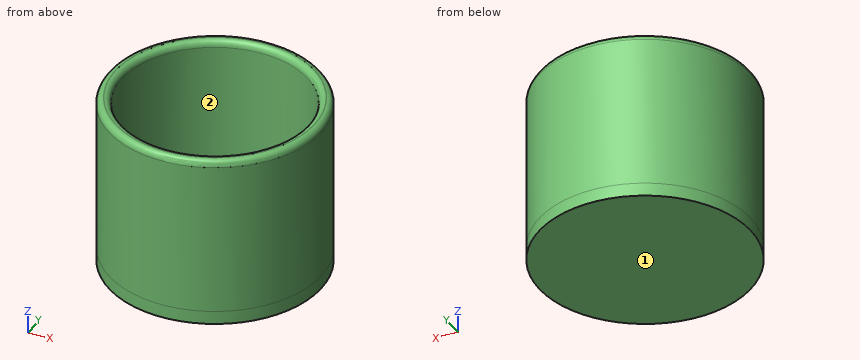
from build123d import *

# Parameters (mm, degrees)
F0_R     = 50.8
F1_DEPTH = 6.35
F2_R     = 50.8
F2_R_2   = 44.45
F3_DEPTH = 76.2
F4_R     = 3.066051
F5_R     = 3.066051


with BuildPart() as f1:
    # F0 (on Top) → F1 (new body)
    with BuildSketch(Plane.XY):
        Circle(F0_R)
    extrude(amount=-F1_DEPTH)

    # F2 (on face) → F3 (join)
    with BuildSketch(Plane.XY):
        Circle(F2_R)
        Circle(F2_R_2, mode=Mode.SUBTRACT)
    extrude(amount=F3_DEPTH)

    # F4
    f4_edges = [f1.edges().sort_by_distance(p)[0] for p in [
        (-50.8, 0, 76.2),
    ]]
    fillet(f4_edges, radius=F4_R)

    # F5
    f5_edges = [f1.edges().sort_by_distance(p)[0] for p in [
        (-44.45, 0, 76.2),
    ]]
    fillet(f5_edges, radius=F5_R)


solid = f1.part
Geometry: final body of the model. Coordinates: model frame, mm. Face numbers are marked on the shaded views. Round coordinates to 2 decimals unless told otherwise and drop trailing zeros. Loops run counter-clockwise (first coordinate to the right, second up) from the corner with the lowest first, then second, coordinate; pieces in that order, holes last. Notation, with made-up numbers: M -30,68.25 L 6,68.25 A23 ccw 6,104.25 Z; hole C -2,24.25 d8. An arc over 180 degrees is marked long. Put each result on its own line as item: value. Start each with the question number.
(1) Draft query along Y for the marked faces 1 and 2. Return one class per face: +Y half, -Y half, draft (parallel to the pull), parting line (faces both ways), or undercut.
(2) Material intervals for line 1 along Y through (x, z) = (0, 43); line 2 along Z through (x, y) = (38, 3); line 3 along Y through (x, z) = (-17.5, 38.5), sorted ascending. Write a range as [from, to].
(3) Section query A-A (x = 0). Return loops of the section in (y, z).
(4) Contact query for flat-ended pins moving along their axis: pin 1 Ø8 at (y, z) = (18.5, 49.5) entering from +X; pin 2 Ø1 at (x, y) = (14, 28) entering from +Z; pin 3 Ø8 at (x, z) = (18, 31) entering from -Y. Output: stop coordinate, or through.
(5) Section query C-C (z = 55.5). Return loops of the section in (x, y).
Findings below:
1. face 1: draft
1. face 2: undercut
2. line 1: y = [-50.8, -44.45], [44.45, 50.8]
2. line 2: z = [-6.35, 0]
2. line 3: y = [-47.69, -40.86], [40.86, 47.69]
3. outline: M -50.8,-6.35 L 50.8,-6.35 L 50.8,73.13 A3.07 ccw 47.73,76.2 L 47.52,76.2 A3.07 ccw 44.45,73.13 L 44.45,0 L -44.45,0 L -44.45,73.13 A3.07 ccw -47.52,76.2 L -47.73,76.2 A3.07 ccw -50.8,73.13 Z
4. pin 1: stops at x = 48.69
4. pin 2: stops at z = 0
4. pin 3: stops at y = -48.83
5. outline: C 0,0 d101.6; hole C 0,0 d88.9
